from build123d import *

# Parameters (mm, degrees)
F2_SIZE = 9.99999
F3_SIZE = 3


# Not quite as in the source:
# - a fillet or chamfer is up to 0.001 mm smaller than in the source, because OpenCascade refuses the exact size


with BuildPart() as f1:
    # F0 (on Top) → F1 (revolve)
    with BuildSketch(Plane.XY):
        Polygon((0, 7.5), (0, 0), (160, 0), (160, 40), (150, 40), (150, 27.5), (25, 27.5), (25, 7.5), align=None)
    revolve(axis=Axis((80, 0, 0), (-1, 0, 0)))

    # F2 (size 10 in the source; OpenCascade refuses exactly that, so slightly less here)
    f2_edges = [f1.edges().sort_by_distance(p)[0] for p in [
        (160, -40, 0),
        (150, -27.5, 0),
    ]]
    chamfer(f2_edges, length=F2_SIZE)

    # F3
    f3_edges = [f1.edges().sort_by_distance(p)[0] for p in [
        (25, -27.5, 0),
    ]]
    chamfer(f3_edges, length=F3_SIZE)


solid = f1.part
Build history of the part. All positions in model axes, mm. A direction names the side the tool comes from. Round coordinates to 2 decimals unless told otherwise and drop trailing zeros. Loops run counter-clockwise (first coordinate to the right, second up) from the corner with the lowest first, then second, coordinate; pieces in that order, holes last. Notation, with made-up numbers: (53.5, -28.5) -> (88.5, -28.5) arc R24 ccw to (88.5, -9.5) -> close; hole circle Ø1 at (25, 4.25). An arc over 180 degrees is marked (long way). Use CSV: the item, a comma, the result in double quotes. Start each with the question number.
Q1. Flat gauge pins, fed straight in: pin 1 Ø12 at (x, z) = (87.5, 16.5) entering from +Y; pin 2 Ø4 at (x, z) = (135.5, 13) entering from -Y; pin 3 Ø1 at (y, z) = (25.5, -26.5) entering from -X. Where does each tip first touch, or does it go through?
Q2. Which spindle directions (+Z, -Z, +X, -X, +Y, -Y) get a long thin tool onto all of the face, cutting with end or side? Do faces 1 (the face through (150, 12, -36)), 2 (the face through (160, 0, 0)). Say none if no direction does.
Q3. Saw through at C-C on x = 48.5. Give the cut face in (y, z), and give its area (3 significant figures).
Q4. Drill centre lines: L1, parallel to X at y = 19, z = -2; L2, parallel to Y at x = 32, z = -1. Where is each one in solid material? Low to high.
Solutions:
1,pin 1,"stops at y = 25.42"
1,pin 2,"stops at y = -25.2"
1,pin 3,"stops at x = 148.78"
2,face 1,"-X"
2,face 2,"+Z, -Z, +X, +Y, -Y"
3,outline,"circle Ø55 at (0, 0)"
3,area,"2,380 mm^2"
4,L1,"x = 25 to 160"
4,L2,"y = -27.48 to 27.48"
